from build123d import *

# Parameters (mm, degrees)
ESQUISSE1_W                  = 150
ESQUISSE1_H                  = 80
BOSS_EXTRU_1_DEPTH           = 5
ESQUISSE2_W                  = 80
ESQUISSE2_H                  = 80
BOSS_EXTRU_2_DEPTH           = 30
ESQUISSE3_W                  = 75
ESQUISSE3_H                  = 80
ENL_V_MAT_EXTRU_1_DEPTH      = 25
ESQUISSE6_R                  = 4
ENL_V_MAT_EXTRU_2_DEPTH      = 40
ESQUISSE7_W                  = 6
ESQUISSE7_H                  = 61
BOSS_EXTRU_3_DEPTH           = 8
ESQUISSE9_W                  = 3
ESQUISSE9_H                  = 50
BOSS_EXTRU_4_DEPTH           = 0.0001
ESQUISSE10_W                 = 3
ESQUISSE10_H                 = 55.5
ENL_V_MAT_EXTRU_3_DEPTH      = 3
ESQUISSE11_W                 = 3
ESQUISSE11_H                 = 55.5
ENL_V_MAT_EXTRU_4_DEPTH      = 3
ESQUISSE12_W                 = 15
ESQUISSE12_H                 = 15
BOSS_EXTRU_5_DEPTH           = 40
BOSS_EXTRU_6_DEPTH           = 1
BOSS_EXTRU_6_DEPTH_BACK      = 7
ESQUISSE13_W                 = 44
ESQUISSE13_H                 = 25
BOSS_EXTRU_7_DEPTH           = 1
BOSS_EXTRU_7_DEPTH_BACK      = 7
ESQUISSE16_W                 = 23
ESQUISSE16_H                 = 12
ENL_V_MAT_EXTRU_5_DEPTH      = 5
ESQUISSE18_W                 = 14.2
ESQUISSE18_H                 = 12
ENL_V_MAT_EXTRU_7_DEPTH      = 5
ESQUISSE19_W                 = 25
ESQUISSE19_H                 = 8
BOSS_EXTRU_8_DEPTH           = 20
ENL_V_MAT_EXTRU_8_DEPTH      = 103.197148685
ESQUISSE21_W                 = 1.984335448
ESQUISSE21_H                 = 3
BOSS_EXTRU_9_DEPTH           = 25
ESQUISSE22_W                 = 3
ESQUISSE22_H                 = 25
BOSS_EXTRU_10_DEPTH          = 75
ESQUISSE23_W                 = 80
ESQUISSE23_H                 = 5
BOSS_EXTRU_11_DEPTH          = 9.96
ESQUISSE24_W                 = 11.416766346
ESQUISSE24_H                 = 16.447883718
BOSS_EXTRU_12_DEPTH          = 3
ENL_V_MAT_EXTRU_9_DEPTH      = 108.658959683
ENL_V_MAT_EXTRU_9_DEPTH_BACK = 108.658959683


with BuildPart() as part:
    # Esquisse1 → Boss.-Extru.1 (new body)
    with BuildSketch(Plane(origin=(0, 0, 0), x_dir=(1, 0, 0), z_dir=(0, 1, 0))):
        Rectangle(ESQUISSE1_W, ESQUISSE1_H)
    extrude(amount=BOSS_EXTRU_1_DEPTH)

    # Esquisse2 → Boss.-Extru.2 (add)
    with BuildSketch(Plane(origin=(0, 5, 0), x_dir=(1, 0, 0), z_dir=(0, 1, 0))):
        with Locations((35, 0)):
            Rectangle(ESQUISSE2_W, ESQUISSE2_H)
    extrude(amount=BOSS_EXTRU_2_DEPTH)

    # Esquisse3 → Enlèv. mat.-Extru.1 (cut)
    with BuildSketch(Plane.XZ):
        with Locations((37.5, 0)):
            Rectangle(ESQUISSE3_W, ESQUISSE3_H)
    extrude(amount=-ENL_V_MAT_EXTRU_1_DEPTH, mode=Mode.SUBTRACT)

    # Esquisse6 → Enlèv. mat.-Extru.2 (cut)
    with BuildSketch(Plane(origin=(0, 35, 0), x_dir=(1, 0, 0), z_dir=(0, 1, 0))):
        with Locations(Location((34.753416048, 0, 0), (0, 0, 270))):
            Circle(ESQUISSE6_R)
    extrude(amount=-ENL_V_MAT_EXTRU_2_DEPTH, mode=Mode.SUBTRACT)

    # Esquisse7 → Boss.-Extru.3 (add)
    with BuildSketch(Plane(origin=(0, 35, 0), x_dir=(1, 0, 0), z_dir=(0, 1, 0))):
        with Locations((-0.015664552, 0)):
            Rectangle(ESQUISSE7_W, ESQUISSE7_H)
        with Locations((70.25575127, 0)):
            Rectangle(ESQUISSE7_W, ESQUISSE7_H)
    extrude(amount=BOSS_EXTRU_3_DEPTH)

    # Esquisse9 → Boss.-Extru.4 (add)
    with BuildSketch(Plane(origin=(0, 5, 0), x_dir=(1, 0, 0), z_dir=(0, 1, 0))):
        Polygon((-27, -36.47894853), (-5, -36.47894853), (-5, -33.47894853), (-24, -33.47894853), (-27, -33.47894853), align=None)
        with Locations((-25.5, -8.47894853)):
            Rectangle(ESQUISSE9_W, ESQUISSE9_H)
    extrude(amount=BOSS_EXTRU_4_DEPTH)

    # Esquisse10 → Enlèv. mat.-Extru.3 (cut)
    with BuildSketch(Plane(origin=(0, 43, 0), x_dir=(1, 0, 0), z_dir=(0, 1, 0))):
        with Locations((1.484335448, 0.25)):
            Rectangle(ESQUISSE10_W, ESQUISSE10_H)
    extrude(amount=-ENL_V_MAT_EXTRU_3_DEPTH, mode=Mode.SUBTRACT)

    # Esquisse11 → Enlèv. mat.-Extru.4 (cut)
    with BuildSketch(Plane(origin=(0, 43, 0), x_dir=(1, 0, 0), z_dir=(0, 1, 0))):
        with Locations((68.75575127, 0.25)):
            Rectangle(ESQUISSE11_W, ESQUISSE11_H)
    extrude(amount=-ENL_V_MAT_EXTRU_4_DEPTH, mode=Mode.SUBTRACT)

    # Esquisse12 → Boss.-Extru.5 (add)
    with BuildSketch(Plane(origin=(0, 5, 0), x_dir=(1, 0, 0), z_dir=(0, 1, 0))):
        with Locations((-67.5, 0)):
            Rectangle(ESQUISSE12_W, ESQUISSE12_H)
    extrude(amount=BOSS_EXTRU_5_DEPTH)

    # Esquisse13 → Boss.-Extru.6 (add, two sides: drawn at the far end of the back side and taken through both)
    with BuildSketch(Plane(origin=(0, 45, 0), x_dir=(1, 0, 0), z_dir=(0, 1, 0)).offset(-BOSS_EXTRU_6_DEPTH_BACK)):
        with Locations((-44.729487472, -0.507142805)):
            Rectangle(ESQUISSE13_W, ESQUISSE13_H)
    extrude(amount=BOSS_EXTRU_6_DEPTH + BOSS_EXTRU_6_DEPTH_BACK)

    # Esquisse14 → Boss.-Extru.7 (add, two sides: drawn at the far end of the back side and taken through both)
    with BuildSketch(Plane(origin=(0, 45, 0), x_dir=(1, 0, 0), z_dir=(0, 1, 0)).offset(-BOSS_EXTRU_7_DEPTH_BACK)):
        Polygon((-66.729487472, -13.007142805), (-75, -7.5), (-75, 7.5), (-66.729487472, 11.992857195), align=None)
    extrude(amount=BOSS_EXTRU_7_DEPTH + BOSS_EXTRU_7_DEPTH_BACK)

    # Esquisse16 → Enlèv. mat.-Extru.5 (cut)
    with BuildSketch(Plane.XZ.offset(-38)):
        with Locations((-40, 1.869279691)):
            Rectangle(ESQUISSE16_W, ESQUISSE16_H)
    extrude(amount=-ENL_V_MAT_EXTRU_5_DEPTH, mode=Mode.SUBTRACT)

    # Esquisse18 → Enlèv. mat.-Extru.7 (cut)
    with BuildSketch(Plane.XZ.offset(-43)):
        with Locations((-35.637534585, 1.827095349)):
            Rectangle(ESQUISSE18_W, ESQUISSE18_H)
    extrude(amount=-ENL_V_MAT_EXTRU_7_DEPTH, mode=Mode.SUBTRACT)

    # Esquisse19 → Boss.-Extru.8 (add)
    with BuildSketch(Plane(origin=(-22.729487472, 0, 0), x_dir=(0, 0, -1), z_dir=(1, 0, 0))):
        with Locations((-0.507142805, 42)):
            Rectangle(ESQUISSE19_W, ESQUISSE19_H)
    extrude(amount=BOSS_EXTRU_8_DEPTH)

    # Esquisse20 → Enlèv. mat.-Extru.8 (cut, through all)
    with BuildSketch(Plane(origin=(0, 0, -11.992857195), x_dir=(-1, 0, 0), z_dir=(0, 0, -1))):
        Polygon((3.015664552, 43), (9.263117513, 46), (2.729487472, 46), (2.729487472, 43), align=None)
    extrude(amount=-ENL_V_MAT_EXTRU_8_DEPTH, mode=Mode.SUBTRACT)

    # Esquisse21 → Boss.-Extru.9 (add)
    with BuildSketch(Plane(origin=(0, 0, -11.992857195), x_dir=(-1, 0, 0), z_dir=(0, 0, -1))):
        with Locations((4.007832276, 36.5)):
            Rectangle(ESQUISSE21_W, ESQUISSE21_H)
    extrude(amount=-BOSS_EXTRU_9_DEPTH)

    # Esquisse22 → Boss.-Extru.10 (add)
    with BuildSketch(Plane(origin=(0, 0, 0), x_dir=(0, 0, -1), z_dir=(1, 0, 0))):
        with Locations((-38.5, 12.5)):
            Rectangle(ESQUISSE22_W, ESQUISSE22_H)
    boss_extru_10 = extrude(amount=BOSS_EXTRU_10_DEPTH)

    # Symétrie1: Boss.-Extru.10 across plane
    add(boss_extru_10.mirror(Plane.XY))

    # Esquisse23 → Boss.-Extru.11 (add)
    with BuildSketch(Plane.ZY.offset(75)):
        with Locations((0, 2.5)):
            Rectangle(ESQUISSE23_W, ESQUISSE23_H)
    extrude(amount=BOSS_EXTRU_11_DEPTH)

    # Esquisse24 → Boss.-Extru.12 (add)
    with BuildSketch(Plane(origin=(0, 5, 4.193760708), x_dir=(1, 0, 0), z_dir=(0, 1, 0))):
        with Locations((-74.621764305, 25.318857606)):
            Rectangle(ESQUISSE24_W, ESQUISSE24_H)
    extrude(amount=BOSS_EXTRU_12_DEPTH)

    # Esquisse25 → Enlèv. mat.-Extru.9 (cut, two sides: drawn at the far end of the back side and taken through both)
    with BuildSketch(Plane.XY.offset(7.5).offset(-ENL_V_MAT_EXTRU_9_DEPTH_BACK)):
        Polygon((-304.628474167, -184.117769245), (-75, 38), (-66.729487472, 46), (162.898986696, 268.117769245), (-281.336551795, 727.37471758), (-748.864012658, 275.139179089), align=None)
    extrude(amount=ENL_V_MAT_EXTRU_9_DEPTH + ENL_V_MAT_EXTRU_9_DEPTH_BACK, mode=Mode.SUBTRACT)


solid = part.part
The listing builds one solid part. Answer for the finished solid, in the listing's coordinates (mm). A direction names the side the tool comes from. Round coordinates to 2 decimals unless told otherwise and drop trailing zeros. Write each loop counter-clockwise with the first axis right and the second up, starting at its lowest first coordinate (ties: lowest second). Pieces come first, ordered by that corner, then holes. Notation, with made-up numbers: (87.25, 73.25) - (112.25, 73.25) arc R31 cw to (112.25, 100.25) - close; hole circle Ø7 at (16.5, -34.5). An arc over 180 degrees is marked (long way). Use one line per item in the form item = value. Start each with the question number.
Item 1: Find the intervals of material crossed by line 1 (X direction, y = 28.25, z = 0); line 2 (Y direction, x = -10, z = -11.5); line 3 (X direction, y = 41.5, z = -12.5), in increasing order. Write a range as [from, to].
Item 2: Flat-ended cylindrical pins translate along their axes: pin 1 Ø0.9 at (x, y) = (-35.5, 44) entering from -Z; pin 2 Ø4 at (y, z) = (25.5, -23.5) entering from -X; pin 3 Ø6 at (x, z) = (3.5, 14.5) entering from -Y. Find the tip coordinate at first contact, or state that the pin passes through.
Item 3: Determine the mould class of faces 1 (the flat face through (-42.738, 44, 2)), 2 (the flat face through (-75, 8, -21)), 3 (the flat face through (-40, 40, -4.131)) for opening direction Y: +Y half, -Y half, draft (parallel to the pull), parting line (faces both ways), or undercut.
Item 4: A cutting plane is placed at D-D (x = 16). Write down the section's boundary in (y, z), plus the area to 3 significant figures.
Item 5: A cutting plane is placed at A-A (x = -36). Write down the section's boundary in (y, z).
Item 6: A cutting plane is placed at C-C (y = 32.5). Write down the section's boundary in (x, z).
Item 7: A tool of negligible diameter and unlimited length cuts with its end or side. For faces 4 (the flat face through (-75, 6, -12.901)), 5 (the flat face through (70, 39, -30.5)), 6 (the flat face through (70.256, 42, 0)), 7 (the flat face through (37, 12, 37)), from which of +Z, -Z, +X, -X, +Y, -Y can it reach the whole face along a straight path? Write none if from no direction.
The answers:
q1.line_1 = [-75, -60], [-5, 30.75], [38.75, 75]
q1.line_2 = [0, 5], [38, 46]
q1.line_3 = [-3.02, -0.02], [70.26, 73.26]
q2.pin_1 = -11.99
q2.pin_2 = -5
q2.pin_3 = 25
q3.face_1 = draft
q3.face_2 = +Y half
q3.face_3 = undercut
q4.outline = (0, -40) - (35, -40) - (35, 40) - (0, 40) - (0, 37) - (25, 37) - (25, -37) - (0, -37) - close
q4.area = 950 mm^2
q5.outline = (0, -40) - (5, -40) - (5, 40) - (0, 40) - close; (38, -11.99) - (46, -11.99) - (46, -4.17) - (43, -4.17) - (43, -4.13) - (38, -4.13) - close; (38, 7.87) - (43, 7.87) - (43, 7.83) - (46, 7.83) - (46, 13.01) - (38, 13.01) - close
q6.outline = (-75, -7.5) - (-60, -7.5) - (-60, 7.5) - (-75, 7.5) - close; (-5, -40) - (75, -40) - (75, 40) - (-5, 40) - close; hole circle Ø8 at (34.75, 0)
q7.face_4 = -X, +Y
q7.face_5 = -Z, +X, -X, +Y
q7.face_6 = +Y
q7.face_7 = +X, -Y
